Verification items for the finished model (mm, model axes). Face numbers are marked on the shaded views. Round coordinates to 2 decimals unless told otherwise and drop trailing zeros. Order: outer loops, then holes, each group sorted by start corner. A loop starts at its lowest first (then second) coordinate and runs counter-clockwise, first axis right, second up. Notation, with made-up numbers: (-9, 6.25) -> (29, 6.25) arc R18 cw to (29, 14.25) -> close; hole circle Ø5 at (-4, 66). An arc over 180 degrees is marked (long way). Put each result on its own line as item: value.
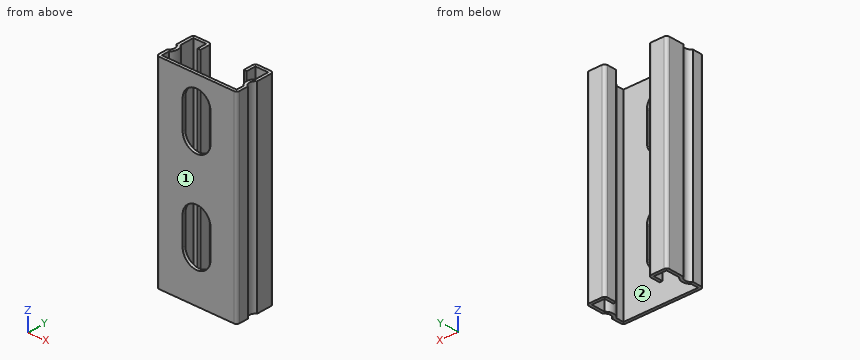
from build123d import *

# Parameters (mm, degrees)
BASE_EXTRUDE_DEPTH = 101.6
SLOT_DEPTH         = 118.113754477
LPATTERN1_COUNT    = 2
LPATTERN1_PITCH    = 50.8


with BuildPart() as part:
    # Sketch1 → Base-Extrude (new body)
    with BuildSketch(Plane.XY):
        with BuildLine():
            Line((-20.6375, 10.4394), (-20.6375, 2.59565134))
            ThreePointArc((-20.6375, 2.59565134), (-19.1389, 0), (-20.6375, -2.59565134))
            Line((-20.6375, -2.59565134), (-20.6375, -7.2136))
            ThreePointArc((-20.6375, -7.2136), (-20.198570222, -8.273270222), (-19.1389, -8.7122))
            Line((-19.1389, -8.7122), (19.1389, -8.7122))
            ThreePointArc((19.1389, -8.7122), (20.198570222, -8.273270222), (20.6375, -7.2136))
            Line((20.6375, -7.2136), (20.6375, -2.59565134))
            ThreePointArc((20.6375, -2.59565134), (19.1389, 0), (20.6375, 2.59565134))
            Line((20.6375, 2.59565134), (20.6375, 10.4394))
            ThreePointArc((20.6375, 10.4394), (20.198570222, 11.499070222), (19.1389, 11.938))
            Line((19.1389, 11.938), (12.6111, 11.938))
            ThreePointArc((12.6111, 11.938), (11.551429778, 11.499070222), (11.1125, 10.4394))
            Line((11.1125, 10.4394), (11.1125, 5.588))
            Line((11.1125, 5.588), (12.6111, 5.588))
            Line((12.6111, 5.588), (12.6111, 10.4394))
            Line((12.6111, 10.4394), (19.1389, 10.4394))
            Line((19.1389, 10.4394), (19.1389, 3.350971471))
            ThreePointArc((19.1389, 3.350971471), (17.6403, 0), (19.1389, -3.350971471))
            Line((19.1389, -3.350971471), (19.1389, -7.2136))
            Line((19.1389, -7.2136), (-19.1389, -7.2136))
            Line((-19.1389, -7.2136), (-19.1389, -3.350971471))
            ThreePointArc((-19.1389, -3.350971471), (-17.6403, 0), (-19.1389, 3.350971471))
            Line((-19.1389, 3.350971471), (-19.1389, 10.4394))
            Line((-19.1389, 10.4394), (-12.6111, 10.4394))
            Line((-12.6111, 10.4394), (-12.6111, 5.588))
            Line((-12.6111, 5.588), (-11.1125, 5.588))
            Line((-11.1125, 5.588), (-11.1125, 10.4394))
            ThreePointArc((-11.1125, 10.4394), (-11.551429778, 11.499070222), (-12.6111, 11.938))
            Line((-12.6111, 11.938), (-19.1389, 11.938))
            ThreePointArc((-19.1389, 11.938), (-20.198570222, 11.499070222), (-20.6375, 10.4394))
        make_face()
    extrude(amount=BASE_EXTRUDE_DEPTH)

    # Sketch2 → Slot (cut, through all)
    with BuildSketch(Plane(origin=(-0.747608536, -8.7122, -11.677878955), x_dir=(1, 0, 0), z_dir=(0, -1, 0))):
        with BuildLine():
            Line((7.891358536, 48.984128955), (7.891358536, 34.696628955))
            ThreePointArc((7.891358536, 34.696628955), (0.747608536, 27.552878955), (-6.396141464, 34.696628955))
            Line((-6.396141464, 34.696628955), (-6.396141464, 48.984128955))
            ThreePointArc((-6.396141464, 48.984128955), (0.747608536, 56.127878955), (7.891358536, 48.984128955))
        make_face()
    slot = extrude(amount=-SLOT_DEPTH, mode=Mode.SUBTRACT)

    # LPattern1: Slot ×2
    with Locations(*[(0, 0, i * LPATTERN1_PITCH) for i in range(1, LPATTERN1_COUNT)]):
        add(slot, mode=Mode.SUBTRACT)


solid = part.part
Item 1: Gauge pin test, flat ends, axial feed: pin 1 Ø1 at (y, z) = (2.5, 33) entering from +X; pin 2 Ø1.2 at (y, z) = (-8, 31.5) entering from -X; pin 3 Ø8 at (x, z) = (1.5, 70) entering from +Y; pin 4 Ø0.7 at (y, z) = (-8.5, 31.5) entering from +X. Record the tip position at first contact, or that the pin passes through.
Check sheet entries:
pin 1: stops at x = 20.64
pin 2: stops at x = -20.63
pin 3: stops at y = -7.21
pin 4: stops at x = 20.31
Item 2: Section check C-C on y = -0.5. Record the boundary of the cut face in (x, z).
Check sheet entries:
outline: (-19.18, 0) -> (-17.67, 0) -> (-17.67, 101.6) -> (-19.18, 101.6) -> close; (17.67, 0) -> (19.18, 0) -> (19.18, 101.6) -> (17.67, 101.6) -> close
Item 3: Section check D-D on x = -14.5. Record the boundary of the cut face in (y, z).
Check sheet entries:
outline: (-8.71, 0) -> (-7.21, 0) -> (-7.21, 101.6) -> (-8.71, 101.6) -> close; (10.44, 0) -> (11.94, 0) -> (11.94, 101.6) -> (10.44, 101.6) -> close
Item 4: Release check for a two-part mould opening along Y. For the marked faces 1 and 2 record: +Y half, -Y half, draft (parallel to the pull), parting line (faces both ways), or undercut.
Check sheet entries:
face 1: -Y half
face 2: undercut
Item 5: Section check A-A on x = 0. Record the boundary of the cut face in (y, z) (3 decimals).
Check sheet entries:
outline: (-8.712, 0) -> (-7.214, 0) -> (-7.214, 15.875) -> (-8.712, 15.875) -> close; (-8.712, 44.45) -> (-7.214, 44.45) -> (-7.214, 66.675) -> (-8.712, 66.675) -> close; (-8.712, 95.25) -> (-7.214, 95.25) -> (-7.214, 101.6) -> (-8.712, 101.6) -> close
Item 6: Material ranges on L1, parallel to X at y = 6.25, z = 75; L2, parallel to Y at x = -14.5, z = 77.5; L3, parallel to X at y = -6.25, z = 31, recorded low to high. Write a range as [from, to].
Check sheet entries:
L1: x = [-20.64, -19.14], [-12.61, -11.11], [11.11, 12.61], [19.14, 20.64]
L2: y = [-8.71, -7.21], [10.44, 11.94]
L3: x = [-20.64, -19.14], [19.14, 20.64]
